Autodesk Inventor part; units mm, degrees
ref_plane "YZ Plane" through (0, 0, 0) normal (1, 0, 0) x (0, 1, 0)
ref_plane "XZ Plane" through (0, 0, 0) normal (0, 1, 0) x (-1, 0, 0)
ref_plane "XY Plane" through (0, 0, 0) normal (0, 0, 1) x (1, 0, 0)
sketch "Sketch1" plane through (0, 0, 0) normal (0, 0, 1) x (1, 0, 0)
  line L0 (-3.2, -3.2) -> (3.2, -3.2)
  line L1 (3.2, -3.2) -> (3.2, 3.2)
  line L2 (3.2, 3.2) -> (-3.2, 3.2)
  line L3 (-3.2, 3.2) -> (-3.2, -3.2)
  line L4 (-3.2, -3.2) -> (3.2, 3.2) construction
  line L5 (3.2, -3.2) -> (-3.2, 3.2) construction
  line L6 (-4.2, 4.2) -> (4.2, 4.2)
  line L7 (4.2, 4.2) -> (4.2, -4.2)
  line L8 (4.2, -4.2) -> (-4.2, -4.2)
  line L9 (-4.2, -4.2) -> (-4.2, 4.2)
  line L10 (-4.2, 4.2) -> (4.2, -4.2) construction
  line L11 (4.2, 4.2) -> (-4.2, -4.2) construction
  line L12 (6.4, -6.4) -> (-6.4, -6.4)
  line L13 (-6.4, -6.4) -> (-6.4, 6.4)
  line L14 (-6.4, 6.4) -> (6.4, 6.4)
  line L15 (6.4, 6.4) -> (6.4, -6.4)
  line L16 (6.4, -6.4) -> (-6.4, 6.4) construction
  line L17 (-6.4, -6.4) -> (6.4, 6.4) construction
  point P0 (0, 0)
  dimension "d0" = 6.4
  dimension "d1" = 6.4
  dimension "d2" = 8.4
  dimension "d3" = 8.4
  dimension "d4" = 12.8
extrude "Extrusion1" add sketch "Sketch1" along normal blind 1 contours L6 L7 L8 L9 | L12 L13 L14 L15
extrude "Extrusion2" add sketch "Sketch1" along normal blind 3.2 from surface at 1 contours L6 L7 L8 L9
extrude "Extrusion3" add sketch "Sketch1" against normal blind 2 from surface at 4.2 contours L3 L2 L1 L0 | L6 L7 L8 L9
properties part number "reset button cover"
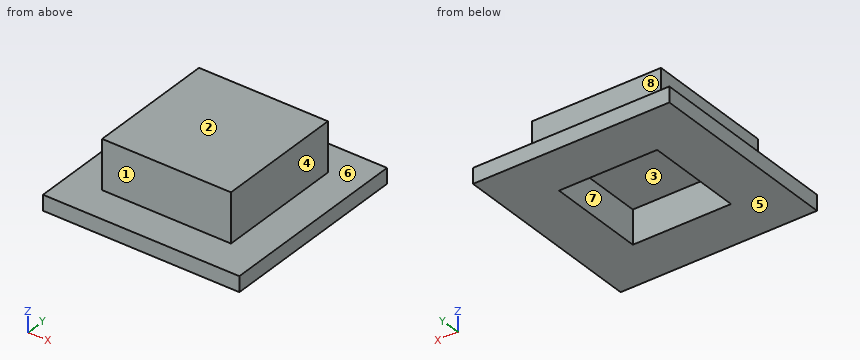
Could you check a few things on this model? Use its own coordinates, in mm. Face numbers are marked on the shaded views. A direction names the side the tool comes from. Give positions to 0.01 mm unless a question says otherwise; leave off trailing zeros. Order: outer loops, then holes, each group sorted by start corner. A loop starts at its lowest first (then second) coordinate and runs counter-clockwise, first axis right, second up. Notation, with made-up numbers: (3, -24.5) -> (32, -24.5) arc R28 cw to (32, 7.5) -> close; hole circle Ø8 at (29, 14). An arc over 180 degrees is marked (long way). Answer in a Markdown table with one row per item. Add a question column.
Item 1: Imagine slicing it at D-D (x = 4). List the corners of the cut face in (y, z) for me, and give its area (3 significant figures).
Item 2: For the marked faces 1, 2, 3, 4 and 5, which set-ups out of +Z, -Z, +X, -X, +Y, -Y let a thin tool reach every point of the face, with its end or its side?
Item 3: Imagine slicing it at B-B (x = -2). List the corners of the cut face in (y, z) for me, and give its area (3 significant figures).
Item 4: We'd pull the mould along Y, two halves only. Please class the marked faces 6, 7 and 8: pulls with the +Y half, pulls with the -Y half, needs draft (parallel to the pull), parting line crosses it, or undercut.
Item 5: I'm going to push flat-ended pins straight in: P1, Ø1, axis at x = 0.5, z = 2.5, coming from the -Y side; P2, Ø7, axis at x = -1, y = -0.5, coming from the -Z side; P3, Ø1.5, axis at y = -2.5, z = 2.5, coming from the -X side; P4, Ø1.5, axis at y = 0.5, z = 3, coming from the +X side. Where does each tip first touch, or does it pass through?
Item 6: Please list where these lines run through material, in increasing order: probe 1 along Y at (x, z) = (-2.25, 0.95); probe 2 along X at (y, z) = (1.25, 1.8).
Item 7: Imagine slicing it at A-A (z = 1.2). List the corners of the cut face in (x, y) for me, and give its area (3 significant figures).
Result:
| question | item | result |
|---|---|---|
| 1 | outline | (-6.4, 0) -> (6.4, 0) -> (6.4, 1) -> (4.2, 1) -> (4.2, 4.2) -> (-4.2, 4.2) -> (-4.2, 1) -> (-6.4, 1) -> close |
| 1 | area | 39.7 mm2 |
| 2 | face 1 | +Z, +X, -X, -Y |
| 2 | face 2 | +Z, +X, -X, +Y, -Y |
| 2 | face 3 | -Z |
| 2 | face 4 | +Z, +X, +Y, -Y |
| 2 | face 5 | -Z, +X, -X, +Y, -Y |
| 3 | outline | (-6.4, 0) -> (-3.2, 0) -> (-3.2, 2.2) -> (3.2, 2.2) -> (3.2, 0) -> (6.4, 0) -> (6.4, 1) -> (4.2, 1) -> (4.2, 4.2) -> (-4.2, 4.2) -> (-4.2, 1) -> (-6.4, 1) -> close |
| 3 | area | 25.6 mm2 |
| 4 | face 6 | needs draft |
| 4 | face 7 | undercut |
| 4 | face 8 | pulls with the +Y half |
| 5 | P1 | y = -4.2 |
| 5 | P2 | z = 0 |
| 5 | P3 | x = -4.2 |
| 5 | P4 | x = 4.2 |
| 6 | probe 1 | -6.4 to -3.2, 3.2 to 6.4 |
| 6 | probe 2 | -4.2 to -3.2, 3.2 to 4.2 |
| 7 | outline | (-4.2, -4.2) -> (4.2, -4.2) -> (4.2, 4.2) -> (-4.2, 4.2) -> close; hole (-3.2, -3.2) -> (3.2, -3.2) -> (3.2, 3.2) -> (-3.2, 3.2) -> close |
| 7 | area | 29.6 mm2 |
